Can you work these out from the model? Positions are in its coordinate system, mm. A direction names the side the tool comes from. Round coordinates to 2 decimals unless told otherwise and drop trailing zeros. Write each loop counter-clockwise with the first axis right and the second up, starting at its lowest first coordinate (ties: lowest second). Pieces come first, ordered by that corner, then holes.
Q1. If we section it at B-B (x = 3.5): Please give me the cut outline in (y, z), plus the area to 3 significant figures.
Q2. If we section it at A-A (y = 4.5): Please give me the cut outline in (x, z), plus the area to 3 significant figures.
Q3. Please list where these lines run through material, in increasing order: line 1 along Z through (x, y) = (-0.5, 5); line 2 along Y through (x, z) = (0, -3.5); line 3 along X through (y, z) = (0, 1.5).
Q4. We'd pull the mould along Y, two halves only. Please class faces 1 (the cylindrical face through (0.52, -2.39, -1.21)), 2 (the cylindrical face through (-2.861, 0.854, -45.631)), 3 (the flat face through (1, 3, -41.564)), 4 (the flat face through (0, -3.797, -14)): +Y half, -Y half, draft (parallel to the pull), parting line (faces both ways), or undercut.
Q5. If we section it at C-C (z = -37): Please give me the cut outline in (x, y), plus the area to 3 significant figures.
Q6. I'm going to push flat-ended pins straight in: pin 1 Ø1.5 at (y, z) = (2.5, -10) entering from -X; pin 2 Ø5 at (x, z) = (0, -7.81) entering from +Y; pin 3 Ø1.1 at (x, y) = (-2, -5) entering from -Z. Where does each tip first touch, or does it pass through?
Q7. For faces 5 (the flat face through (0, -5, -4.814)), 6 (the flat face through (0, 5, -4.814)), 7 (the cylindrical face through (-0.49, 2.59, -5.62)), which set-ups out of +Z, -Z, +X, -X, +Y, -Y let a thin tool reach every point of the face, with its end or its side?
from build123d import *

# Parameters (mm, degrees)
SKETCH1_R                      = 4
BOSS_EXTRUDE2_DEPTH            = 34
SKETCH2_R                      = 2
BOSS_EXTRUDE3_DEPTH            = 6
CHAMFER1_SIZE                  = 0.5
F_3_2_3_2_DIAMETER_HOLE1_D     = 3.2
F_3_2_3_2_DIAMETER_HOLE1_DEPTH = 14
F_3_2_3_2_DIAMETER_HOLE1_TIP   = 0.96137699
CUT_EXTRUDE1_DEPTH             = 41.398019753
CUT_EXTRUDE1_DEPTH_BACK        = 41.398019753
SKETCH5_W                      = 12
SKETCH5_H                      = 1.5
SKETCH5_W_2                    = 4
F_3_0_3_DIAMETER_HOLE1_REACH   = 42.722
F_3_0_3_DIAMETER_HOLE1_BORE_R  = 1.5
SCALE1_SCALE                   = 1.5


with BuildPart() as part:
    # Sketch1 → Boss-Extrude2 (new body)
    with BuildSketch(Plane.XY):
        Circle(SKETCH1_R)
    extrude(amount=-BOSS_EXTRUDE2_DEPTH)

    # Sketch2 → Boss-Extrude3 (add)
    with BuildSketch(Plane(origin=(0, 0, -34), x_dir=(-1, 0, 0), z_dir=(0, 0, -1))):
        Circle(SKETCH2_R)
    extrude(amount=BOSS_EXTRUDE3_DEPTH)

    # Chamfer1
    chamfer1_edges = [part.edges().sort_by_distance(p)[0] for p in [
        (2, 0, -40),
    ]]
    chamfer(chamfer1_edges, length=CHAMFER1_SIZE)

    # Ø3.2 (3.2) Diameter Hole1
    with Locations(Plane.XY):
        with Locations((0, 0)):
            Hole(F_3_2_3_2_DIAMETER_HOLE1_D / 2, depth=F_3_2_3_2_DIAMETER_HOLE1_DEPTH)
            with Locations((0, 0, -(F_3_2_3_2_DIAMETER_HOLE1_DEPTH + F_3_2_3_2_DIAMETER_HOLE1_TIP / 2))):  # 118° drill point
                Cone(0, F_3_2_3_2_DIAMETER_HOLE1_D / 2, F_3_2_3_2_DIAMETER_HOLE1_TIP, mode=Mode.SUBTRACT)

    # Sketch5 → Cut-Extrude1 (cut, two sides: drawn at the far end of the back side and taken through both)
    with BuildSketch(Plane(origin=(0, 0, 0), x_dir=(0, 0, -1), z_dir=(1, 0, 0)).offset(-CUT_EXTRUDE1_DEPTH_BACK)):
        with Locations((15.5, -3.25)):
            Rectangle(SKETCH5_W, SKETCH5_H)
        with Locations((11.5, 3.25)):
            Rectangle(SKETCH5_W_2, SKETCH5_H)
    extrude(amount=CUT_EXTRUDE1_DEPTH + CUT_EXTRUDE1_DEPTH_BACK, mode=Mode.SUBTRACT)

    # Ø3.0 (3) Diameter Hole1 bore → Ø3.0 (3) Diameter Hole1 (cut, up to next)
    with BuildSketch(Plane(origin=(0, 2.5, 0), x_dir=(1, 0, 0), z_dir=(0, 1, 0)), mode=Mode.PRIVATE) as f_3_0_3_diameter_hole1_sk1:
        with Locations((0, 11.5)):
            Circle(F_3_0_3_DIAMETER_HOLE1_BORE_R)
    f_3_0_3_diameter_hole1_tool1 = extrude(f_3_0_3_diameter_hole1_sk1.sketch, amount=-F_3_0_3_DIAMETER_HOLE1_REACH, mode=Mode.PRIVATE) & part.part
    add(f_3_0_3_diameter_hole1_tool1.solids().sort_by_distance((0, 2.5, -11.5))[0], mode=Mode.SUBTRACT)


with BuildPart() as part_1:
    # Scale1: scaled about (4.68e-07, 0.094714404, -18.871986745)
    add(part.part.scale(SCALE1_SCALE).moved(Location((-2.34e-07, -0.047357202, 9.435993373))))


solid = part_1.part
A:
1. outline: (-4.92, -41.56) - (4.83, -41.56) - (4.83, -10.81) - (3.7, -10.81) - (3.7, -4.81) - (4.83, -4.81) - (4.83, 9.44) - (-4.92, 9.44) - (-4.92, -4.81) - (-3.8, -4.81) - (-3.8, -22.81) - (-4.92, -22.81) - close
1. area: 470 mm2
2. outline: (-3.91, -41.56) - (3.91, -41.56) - (3.91, -10.81) - (-3.91, -10.81) - close; (-3.91, -4.81) - (3.91, -4.81) - (3.91, 9.44) - (-3.91, 9.44) - close
2. area: 352 mm2
3. line 1: z = -41.56 to -10.81, -4.81 to 9.44
3. line 2: y = -6.05 to -2.45, 2.35 to 5.95
3. line 3: x = -6 to -2.4, 2.4 to 6
4. face 1: undercut
4. face 2: parting line
4. face 3: draft
4. face 4: -Y half
5. outline: circle Ø12 at (0, -0.05)
5. area: 113 mm2
6. pin 1: stops at x = -5.72
6. pin 2: stops at y = 3.7
6. pin 3: stops at z = -41.56
7. face 5: +X, -X, -Y
7. face 6: +X, -X, +Y
7. face 7: +Y
